Verification items for the finished model (mm, model axes). Round coordinates to 2 decimals unless told otherwise and drop trailing zeros. Order: outer loops, then holes, each group sorted by start corner. A loop starts at its lowest first (then second) coordinate and runs counter-clockwise, first axis right, second up. Notation, with made-up numbers: (-18.5, 9.25) -> (-11.5, 9.25) arc R21 ccw to (-11.5, 41.25) -> close; hole circle Ø8 at (76.5, 43). An arc over 180 degrees is marked (long way). Answer in a Markdown table with one row per item. Add a question column.
```python
from build123d import *

# Parameters (mm, degrees)
SKETCH2_R           = 20
BOSS_EXTRUDE1_DEPTH = 275
SKETCH5_W           = 5
SKETCH5_H           = 9
CUT_EXTRUDE2_DEPTH  = 8
SKETCH8_W           = 4
SKETCH8_H           = 9
CUT_EXTRUDE3_DEPTH  = 4
CUT_EXTRUDE4_START  = 5
SKETCH8_4_W         = 4
SKETCH8_4_H         = 9
CUT_EXTRUDE4_DEPTH  = 4
SKETCH9_W           = 4
SKETCH9_H           = 13
CUT_EXTRUDE5_DEPTH  = 4
CUT_EXTRUDE6_START  = 9
CUT_EXTRUDE6_DEPTH  = 4
SKETCH10_R          = 4.5
CUT_EXTRUDE7_DEPTH  = 277.450718936
CIRPATTERN1_COUNT   = 4


with BuildPart() as part:
    # Sketch2 → Boss-Extrude1 (new body)
    with BuildSketch(Plane.XY):
        Circle(SKETCH2_R)
    extrude(amount=BOSS_EXTRUDE1_DEPTH)

    # Sketch5 → Cut-Extrude2 (cut)
    with BuildSketch(Plane.ZY.offset(20)):
        with Locations((13.5, 0)):
            Rectangle(SKETCH5_W, SKETCH5_H)
    extrude(amount=-CUT_EXTRUDE2_DEPTH, mode=Mode.SUBTRACT)

    # Sketch8 → Cut-Extrude3 (cut)
    with BuildSketch(Plane.XY.offset(11)):
        with Locations((-14, 0)):
            Rectangle(SKETCH8_W, SKETCH8_H)
    extrude(amount=-CUT_EXTRUDE3_DEPTH, mode=Mode.SUBTRACT)

    # Sketch8<4> → Cut-Extrude4 (cut)
    with BuildSketch(Plane.XY.offset(11).offset(CUT_EXTRUDE4_START)):
        with Locations((-14, 0)):
            Rectangle(SKETCH8_4_W, SKETCH8_4_H)
    extrude(amount=CUT_EXTRUDE4_DEPTH, mode=Mode.SUBTRACT)

    # Sketch9 → Cut-Extrude5 (cut)
    with BuildSketch(Plane.XZ.offset(-4.5)):
        with Locations((-14, 13.5)):
            Rectangle(SKETCH9_W, SKETCH9_H)
    extrude(amount=-CUT_EXTRUDE5_DEPTH, mode=Mode.SUBTRACT)

    # Sketch9<2> → Cut-Extrude6 (cut)
    with BuildSketch(Plane.XZ.offset(-4.5).offset(CUT_EXTRUDE6_START)):
        Polygon((-16, 16), (-16, 11), (-16, 7), (-12, 7), (-12, 20), (-16, 20), align=None)
    extrude(amount=CUT_EXTRUDE6_DEPTH, mode=Mode.SUBTRACT)

    # Sketch10 → Cut-Extrude7 (cut, through all)
    with BuildSketch(Plane(origin=(0, 0, 0), x_dir=(-1, 0, 0), z_dir=(0, 0, -1))):
        Circle(SKETCH10_R)
    extrude(amount=-CUT_EXTRUDE7_DEPTH, mode=Mode.SUBTRACT)

    # Sketch13 → Ø3.0 (3) Diameter Hole1 (revolve, cut)
    with BuildSketch(Plane(origin=(-3.955313085, 9.672538364, 275), x_dir=(0, -1, 0), z_dir=(1, 0, 0))):
        Polygon((0, 0), (0, 5.901290929), (1.5, 5), (1.5, 0), align=None)
    f_3_0_3_diameter_hole1 = revolve(axis=Axis((-3.955313085, 9.672538364, 281.35), (0, 0, -1)), mode=Mode.SUBTRACT)

    # CirPattern1: Ø3.0 (3) Diameter Hole1 ×4 about axis
    cirpattern1_axis = Axis((0, 0, 0), (0, 0, 1))
    for i in range(1, CIRPATTERN1_COUNT):
        add(f_3_0_3_diameter_hole1.rotate(cirpattern1_axis, i * 360 / CIRPATTERN1_COUNT), mode=Mode.SUBTRACT)


solid = part.part
```
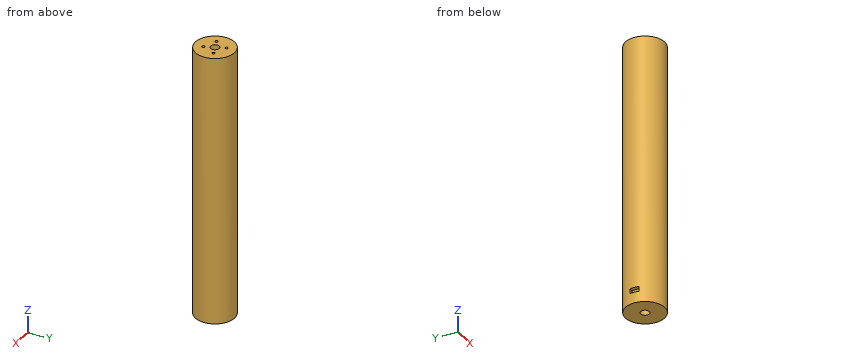
1) Thickness scan on L1, parallel to Y at x = 0, z = 58; L2, parallel to Z at x = -13, y = 1; L3, parallel to X at y = -2, z = 184. Record the ranges inside material, lowest first. Write a range as [from, to].
2) Cross-section at B-B, the plane x = 0. Record the boundary of the cut face in (y, z).
3) Cross-section at D-D, the plane y = -17. Record the boundary of the cut face in (x, z).
4) Cross-section at A-A, the plane y = 0. Record the boundary of the cut face in (x, z), and give its area (3 significant figures).
5) Cross-section at C-C, the plane z = 178. Record the boundary of the cut face in (x, y), and give its area (3 significant figures).
6) Depth check by flat-ended pin: P1, Ø8, axis at x = 4.5, z = 69.5, coming from the +Y side; P2, Ø4.5, axis at x = -14.5, z = 11.5, coming from the -Y side; P3, Ø4, axis at x = 0.5, z = 37.5, coming from the -Y side. Enter the tip coordinate at first touch or a pass-through.
Results below:
| question | item | result |
|---|---|---|
| 1 | L1 | [-20, -4.5], [4.5, 20] |
| 1 | L2 | [0, 7], [20, 275] |
| 1 | L3 | [-19.9, -4.03], [4.03, 19.9] |
| 2 | outline | (-20, 0) -> (-4.5, 0) -> (-4.5, 275) -> (-20, 275) -> close; (4.5, 0) -> (20, 0) -> (20, 275) -> (4.5, 275) -> close |
| 3 | outline | (-10.54, 0) -> (10.54, 0) -> (10.54, 275) -> (-10.54, 275) -> close |
| 4 | outline | (-20, 0) -> (-4.5, 0) -> (-4.5, 275) -> (-20, 275) -> (-20, 16) -> (-16, 16) -> (-16, 20) -> (-12, 20) -> (-12, 7) -> (-16, 7) -> (-16, 11) -> (-20, 11) -> close; (4.5, 0) -> (20, 0) -> (20, 275) -> (4.5, 275) -> close |
| 4 | area | 8,450 mm² |
| 5 | outline | circle Ø40 at (0, 0); hole circle Ø9 at (0, 0) |
| 5 | area | 1,190 mm² |
| 6 | P1 | y = 19.99 |
| 6 | P2 | y = -15.81 |
| 6 | P3 | y = -20 |
